from build123d import *

# Parameters (mm, degrees)
SKETCH_3_R               = 3.3
CUT_EXTRUDE_1_DEPTH      = 6
SKETCH_4_R               = 3.3
CUT_EXTRUDE_2_DEPTH      = 6
SKETCH_5_R               = 3.3
CUT_EXTRUDE_3_DEPTH      = 6
SKETCH_6_R               = 3.3
CUT_EXTRUDE_4_DEPTH      = 6
CUT_EXTRUDE_5_DEPTH      = 42
CUT_EXTRUDE_5_DEPTH_BACK = 42
SKETCH_7_W               = 40
SKETCH_7_H               = 32
CUT_EXTRUDE_6_DEPTH      = 42
CUT_EXTRUDE_6_DEPTH_BACK = 42
SKETCH_8_W               = 40
SKETCH_8_H               = 32


with BuildPart() as part:
    # Sketch 1 → Revolve 1 (revolve)
    with BuildSketch(Plane.XY, mode=Mode.PRIVATE) as revolve_1_sk:
        with BuildLine():
            Line((0, 0), (0, 27.5))
            Line((0, 27.5), (0.5, 28))
            Line((0.5, 28), (5.5, 28))
            Line((5.5, 28), (6, 27.5))
            Line((6, 27.5), (6, 16.5))
            ThreePointArc((6, 16.5), (6.146446609, 16.146446609), (6.5, 16))
            Line((6.5, 16), (39.5, 16))
            Line((39.5, 16), (40, 15.5))
            Line((40, 15.5), (40, 0))
            Line((40, 0), (0, 0))
        make_face()
    revolve(revolve_1_sk.sketch.rotate(Axis((40, 0, 0), (-1, 0, 0)), 270), axis=Axis((40, 0, 0), (-1, 0, 0)))

    # Sketch 2 → Cut-Revolve 1 (revolve, cut)
    with BuildSketch(Plane.XY, mode=Mode.PRIVATE) as cut_revolve_1_sk:
        Polygon((0, 0), (0, 10), (2, 8), (38, 8), (40, 10), (40, 0), align=None)
    revolve(cut_revolve_1_sk.sketch.rotate(Axis((40, 0, 0), (-1, 0, 0)), 270), axis=Axis((40, 0, 0), (-1, 0, 0)), mode=Mode.SUBTRACT)

    # Sketch 3 → Cut-Extrude 1 (cut)
    with BuildSketch(Plane(origin=(0, 0, 0), x_dir=(0, 0, -1), z_dir=(1, 0, 0))):
        with Locations((21, 0)):
            Circle(SKETCH_3_R)
    extrude(amount=CUT_EXTRUDE_1_DEPTH, mode=Mode.SUBTRACT)

    # Sketch 4 → Cut-Extrude 2 (cut)
    with BuildSketch(Plane(origin=(0, 0, 0), x_dir=(0, 0, -1), z_dir=(1, 0, 0))):
        with Locations((-21, 0)):
            Circle(SKETCH_4_R)
    extrude(amount=CUT_EXTRUDE_2_DEPTH, mode=Mode.SUBTRACT)

    # Sketch 5 → Cut-Extrude 3 (cut)
    with BuildSketch(Plane(origin=(0, 0, 0), x_dir=(0, 0, -1), z_dir=(1, 0, 0))):
        with Locations((0, 21)):
            Circle(SKETCH_5_R)
    extrude(amount=CUT_EXTRUDE_3_DEPTH, mode=Mode.SUBTRACT)

    # Sketch 6 → Cut-Extrude 4 (cut)
    with BuildSketch(Plane(origin=(0, 0, 0), x_dir=(0, 0, -1), z_dir=(1, 0, 0))):
        with Locations((0, -21)):
            Circle(SKETCH_6_R)
    extrude(amount=CUT_EXTRUDE_4_DEPTH, mode=Mode.SUBTRACT)

    # Sketch 7 → Cut-Extrude 5 (cut, two sides: drawn at the far end of the back side and taken through both)
    with BuildSketch(Plane.XY.offset(-CUT_EXTRUDE_5_DEPTH_BACK)):
        with Locations((20, 32)):
            Rectangle(SKETCH_7_W, SKETCH_7_H)
    extrude(amount=CUT_EXTRUDE_5_DEPTH + CUT_EXTRUDE_5_DEPTH_BACK, mode=Mode.SUBTRACT)

    # Sketch 8 → Cut-Extrude 6 (cut, two sides: drawn at the far end of the back side and taken through both)
    with BuildSketch(Plane.XY.offset(-CUT_EXTRUDE_6_DEPTH_BACK)):
        with Locations((20, -32)):
            Rectangle(SKETCH_8_W, SKETCH_8_H)
    extrude(amount=CUT_EXTRUDE_6_DEPTH + CUT_EXTRUDE_6_DEPTH_BACK, mode=Mode.SUBTRACT)


solid = part.part
Model file for the job. Use its own axes, mm. A direction names the side the tool comes from. Round coordinates to 2 decimals unless told otherwise and drop trailing zeros. Order: outer loops, then holes, each group sorted by start corner. A loop starts at its lowest first (then second) coordinate and runs counter-clockwise, first axis right, second up.
(1) Band-saw the part on A-A (y = 0). Give the number of separate pieces and of enclosed holes in the cut face, then the cut area to 3 significant figures.
(2) Band-saw the part on C-C (x = 28.5). List the corners of the cut face in (y, z), then the cut area to 3 significant figures.
(3) Band-saw the part on B-B (z = 21). List the corners of the cut face in (x, y), then the cut area to 3 significant figures.
(4) 3-axis set-ups, long thin cutter, end or side, ignore diameter. For faces 1 (the face through (3, 16, 0)), 2 (the face through (6, 4, -19)), 3 (the face through (6, -3, 18)): which of +Z, -Z, +X, -X, +Y, -Y reach the whole face in a straight line?
(5) Pull direction Z, two halves, no side cores. Call faces 4 (the face through (23.23, -15.62, -3.47)), 5 (the face through (5.865, 0.24, -27.634)), 6 (the face through (2.96, -1.26, 17.95)), 7 (the face through (0.14, -0.24, 27.64)): released by +Z, released by -Z, zero draft, split by the parting line, or undercut.
(6) Drill centre lines: line 1 (Y direction, x = 1, z = -21); line 2 (X direction, y = -11.5, z = 17); line 3 (Y direction, x = 19, z = 7). Where is each one in solid material? Low to high.
(7) Pin check, flat tips, straight feed: pin 1 (1 mm diameter, centred on y = 5, z = 4.5, fed in from +X); pin 2 (5 mm diameter, centred on x = 14.5, y = -3, fed in from -Z); pin 3 (7.5 mm diameter, centred on y = 0, z = -21, fed in from -X); pin 4 (8 mm diameter, centred on x = 8, y = 2.5, fed in from +Z). Stop position of each tip, or through.
Verdict:
1. separate pieces: 4
1. enclosed holes: 0
1. area: 696 mm2
2. outline: circle Ø32 at (0, 0); hole circle Ø16 at (0, 0)
2. area: 603 mm2
3. outline: (0, -16) - (6, -16) - (6, -3.3) - (0, -3.3) - close; (0, 3.3) - (6, 3.3) - (6, 16) - (0, 16) - close
3. area: 152 mm2
4. face 1: +Z, -Z, +X, -X, +Y
4. face 2: -Z, +X
4. face 3: +Z, +X
5. face 4: split by the parting line
5. face 5: released by -Z
5. face 6: undercut
5. face 7: released by +Z
6. line 1: y = -16 to -3.3, 3.3 to 16
6. line 2: x = 0 to 6
6. line 3: y = -14.39 to -3.87, 3.87 to 14.39
7. pin 1: passes through
7. pin 2: stops at z = -15.99
7. pin 3: stops at x = 0
7. pin 4: stops at z = 28
